from build123d import *

# Parameters (mm, degrees)
SKETCH_1_R      = 2
EXTRUDE_1_DEPTH = 5


with BuildPart() as part:
    # 草图1 → 凸台-拉伸1 (new body)
    with BuildSketch(Plane.XY):
        with BuildLine():
            Line((-110, 147.74), (-88.912084744, 0))
            Line((-88.912084744, 0), (88.912084744, 0))
            Line((88.912084744, 0), (110, 147.74))
            ThreePointArc((110, 147.74), (99.541573939, 165.317211576), (79.104163323, 164.511426389))
            Line((79.104163323, 164.511426389), (5.447918339, 116.65941923))
            ThreePointArc((5.447918339, 116.65941923), (0, 115.045132425), (-5.447918339, 116.65941923))
            Line((-5.447918339, 116.65941923), (-79.104163323, 164.511426389))
            ThreePointArc((-79.104163323, 164.511426389), (-99.541573939, 165.317211576), (-110, 147.74))
        make_face()
        with Locations((61.7, 105.973140904)):
            Circle(SKETCH_1_R, mode=Mode.SUBTRACT)
        with Locations((-61.7, 21.473140904)):
            Circle(SKETCH_1_R, mode=Mode.SUBTRACT)
        with Locations((-61.7, 39.973140904)):
            Circle(SKETCH_1_R, mode=Mode.SUBTRACT)
        with Locations((-26.5, 16.7)):
            Circle(SKETCH_1_R, mode=Mode.SUBTRACT)
        with Locations((-8, 16.7)):
            Circle(SKETCH_1_R, mode=Mode.SUBTRACT)
        with Locations((8, 16.7)):
            Circle(SKETCH_1_R, mode=Mode.SUBTRACT)
        with Locations((26.5, 16.7)):
            Circle(SKETCH_1_R, mode=Mode.SUBTRACT)
        with Locations((-61.7, 87.473140904)):
            Circle(SKETCH_1_R, mode=Mode.SUBTRACT)
        with Locations((-61.7, 105.973140904)):
            Circle(SKETCH_1_R, mode=Mode.SUBTRACT)
        with Locations((-90, 147.74)):
            Circle(SKETCH_1_R, mode=Mode.SUBTRACT)
        with Locations((0, 89.27)):
            Circle(SKETCH_1_R, mode=Mode.SUBTRACT)
        with Locations((90, 147.74)):
            Circle(SKETCH_1_R, mode=Mode.SUBTRACT)
        with Locations((61.7, 87.473140904)):
            Circle(SKETCH_1_R, mode=Mode.SUBTRACT)
        with Locations((61.7, 39.973140904)):
            Circle(SKETCH_1_R, mode=Mode.SUBTRACT)
        with Locations((61.7, 21.473140904)):
            Circle(SKETCH_1_R, mode=Mode.SUBTRACT)
    extrude(amount=EXTRUDE_1_DEPTH)


solid = part.part
For this review, take the finished solid that the model builds, in its own axes (mm). A direction names the side the tool comes from. Coordinates: 2 decimals unless noted, no trailing zeros. Loops run counter-clockwise (first coordinate to the right, second up) from the corner with the lowest first, then second, coordinate; pieces in that order, holes last. Notation, with made-up numbers: (69.25, 69.25) - (112.25, 69.25) arc R20 cw to (112.25, 89.25) - close; hole circle Ø1 at (-30, -22.5). An arc over 180 degrees is marked (long way). Return JSON: item names as keys, results as strings.
Item 1: For faces 1 (the flat face through (-2, 85, 5)), 2 (the flat face through (-41.76, 140.25, 2.46)), list the 3-axis set-ups (+Z, -Z, +X, -X, +Y, -Y) from which the entire face can be reached by the end or side of a thin tool; tool diameter is ignored.
Determined:
{"face 1": "+Z, +X, -X, +Y, -Y", "face 2": "+Z, -Z, +Y"}
Item 2: Take a section at A-A (z = 2). State how many separate pieces and enclosed holes the cut face has, then the cut area to 3 significant figures.
Determined:
{"separate pieces": "1", "enclosed holes": "15", "area": "28,800 mm2"}
Item 3: Mouldability with a two-part tool opening along X and no side actions: class faces 3 (the flat face through (99.31, 72.84, 2.46)), 4 (the cylindrical face through (99.805, 165.172, 2.465)), 5 (the flat face through (-99.604, 74.904, 2.465)), 6 (the flat face through (-1, 0, 2)) as pulls with the +X half, pulls with the -X half, needs draft (parallel to the pull), parting line crosses it, or undercut.
Determined:
{"face 3": "pulls with the +X half", "face 4": "undercut", "face 5": "pulls with the -X half", "face 6": "needs draft"}
Item 4: Take a section at C-C (y = 11). Give the boundary of the cut face in (x, z), then the cut area to 3 significant figures.
Determined:
{"outline": "(-90.48, 0) - (90.48, 0) - (90.48, 5) - (-90.48, 5) - close", "area": "905 mm2"}
Item 5: Insertion check: pin 1 (3.5 mm diameter, centred on x = 61.7, y = 105.97, fed in from -Z); pin 2 (1 mm diameter, centred on y = 92, z = 3, fed in from -X); pin 3 (3 mm diameter, centred on y = 64, z = 3, fed in from +X). Each pin has a flat end and moves straight along its axis. Give the tip position at first contact, or say it passes through.
Determined:
{"pin 1": "passes through", "pin 2": "stops at x = -102.12", "pin 3": "stops at x = 98.26"}
Item 6: For line 1 (Y direction, x = 61.7, z = 1.55); line 2 (X direction, y = 18, z = 4); line 3 (X direction, y = 149.5, z = 1.25), list the stretches that pass through material, from the lowest coordinate up.
Determined:
{"line 1": "y = 0 to 19.47, 23.47 to 37.97, 41.97 to 85.47, 89.47 to 103.97, 107.97 to 153.2", "line 2": "x = -91.48 to -28.02, -24.98 to -9.52, -6.48 to 6.48, 9.52 to 24.98, 28.02 to 91.48", "line 3": "x = -109.92 to -90.95, -89.05 to -56, 56 to 89.05, 90.95 to 109.92"}
Item 7: Take a section at B-B (x = -95.5). Give the boundary of the cut face in (y, z), then the cut area to 3 significant figures.
Determined:
{"outline": "(46.15, 0) - (166.97, 0) - (166.97, 5) - (46.15, 5) - close", "area": "604 mm2"}
